from build123d import *

# Parameters (mm, degrees)
BOSS_EXTRUDE1_DEPTH     = 30
BOSS_EXTRUDE2_DEPTH     = 17
SKETCH2_R               = 2
CUT_EXTRUDE7_DEPTH      = 26.5000001
CUT_EXTRUDE2_START      = -17
SKETCH3_R               = 4
CUT_EXTRUDE2_DEPTH      = 9.5000001
CUT_EXTRUDE3_DEPTH      = 31.0000001
CUT_EXTRUDE8_DEPTH      = 6.5
CUT_EXTRUDE8_DEPTH_BACK = 5.6
CHAMFER1_SIZE           = 0.3


with BuildPart() as part:
    # Sketch1 → Boss-Extrude1 (new body)
    with BuildSketch(Plane.XY):
        with BuildLine():
            Line((-9, -10.5), (9, -10.5))
            Line((9, -10.5), (15, -10.5))
            Line((15, -10.5), (15, 0))
            ThreePointArc((15, 0), (0, 15), (-15, 0))
            Line((-15, 0), (-15, -10.5))
            Line((-15, -10.5), (-9, -10.5))
        make_face()
    extrude(amount=BOSS_EXTRUDE1_DEPTH)

    # Sketch4 → Boss-Extrude2 (add)
    with BuildSketch(Plane.XZ.offset(10.5)):
        with BuildLine():
            Line((-12.55, 27.5), (-12.55, 19.5))
            ThreePointArc((-12.55, 19.5), (-16.55, 23.5), (-12.55, 27.5))
        make_face()
        with BuildLine():
            Line((12.55, 2.5), (12.55, 10.5))
            ThreePointArc((12.55, 10.5), (16.55, 6.5), (12.55, 2.5))
        make_face()
    extrude(amount=-BOSS_EXTRUDE2_DEPTH)

    # Sketch2 → Cut-Extrude7 (cut, through all)
    with BuildSketch(Plane.XZ.offset(10.5)):
        with Locations((12.55, 6.5)):
            Circle(SKETCH2_R)
        with Locations((-12.55, 23.5)):
            Circle(SKETCH2_R)
    extrude(amount=-CUT_EXTRUDE7_DEPTH, mode=Mode.SUBTRACT)

    # Sketch3 → Cut-Extrude2 (cut, through all)
    with BuildSketch(Plane.XZ.offset(10.5).offset(CUT_EXTRUDE2_START)):
        with Locations((12.55, 6.5)):
            Circle(SKETCH3_R)
        with Locations((-12.55, 23.5)):
            Circle(SKETCH3_R)
    extrude(amount=-CUT_EXTRUDE2_DEPTH, mode=Mode.SUBTRACT)

    # Sketch5 → Cut-Extrude3 (cut, through all)
    with BuildSketch(Plane.XY.offset(30)):
        with BuildLine():
            Line((-9, -10.5), (9, -10.5))
            Line((9, -10.5), (9, -5.6))
            ThreePointArc((9, -5.6), (0, 10.6), (-9, -5.6))
            Line((-9, -5.6), (-9, -10.5))
        make_face()
    extrude(amount=-CUT_EXTRUDE3_DEPTH, mode=Mode.SUBTRACT)

    # Sketch6 → Cut-Extrude8 (cut, two sides)
    with BuildSketch(Plane(origin=(0, 0, 0), x_dir=(1, 0, 0), z_dir=(0, 1, 0))) as cut_extrude8_sk:
        Polygon((0, -24.914213562), (0, -21.5), (-12.55, -21.5), (-13.964213562, -24.914213562), (-9, -29.878427125), align=None)
        Polygon((0, -7.914213562), (0, -4.5), (12.55, -4.5), (13.964213562, -7.914213562), (9, -12.878427125), align=None)
    extrude(amount=CUT_EXTRUDE8_DEPTH, mode=Mode.SUBTRACT)
    extrude(cut_extrude8_sk.sketch, amount=-CUT_EXTRUDE8_DEPTH_BACK, mode=Mode.SUBTRACT)

    # Chamfer1
    chamfer1_edges = [part.edges().sort_by_distance(p)[0] for p in [
        (0, 15, 0),
        (15, -5.25, 0),
        (-12, -10.5, 0),
        (-15, -5.25, 0),
        (12, -10.5, 0),
        (0, 10.6, 0),
        (9, -8.05, 0),
        (-9, -8.05, 0),
    ]]
    chamfer(chamfer1_edges, length=CHAMFER1_SIZE)


solid = part.part
Verification items for the finished model (mm, model axes). A direction names the side the tool comes from. Round coordinates to 2 decimals unless told otherwise and drop trailing zeros. Loops run counter-clockwise (first coordinate to the right, second up) from the corner with the lowest first, then second, coordinate; pieces in that order, holes last. Notation, with made-up numbers: (84, 59.5) - (109, 59.5) arc R29 cw to (109, 98.5) - close; hole circle Ø2 at (40, 33.25). An arc over 180 degrees is marked (long way). Use one line per item in the form item = value.
1. Scan lines: probe 1 along X at (y, z) = (-8.5, 19); probe 2 along Y at (x, z) = (12, 13); probe 3 along X at (y, z) = (-3, 6.5). Record each from-to range of solid material in increasing order.
A:
probe_1 = -15 to -9, 9 to 15
probe_2 = -10.5 to 9
probe_3 = -15 to -10.17, 14.55 to 16.55
2. Access from +Z, -Z, +X, -X, +Y, -Y to the whole of each face (thin tool, end or side, straight path). Record for faces 4 (the flat face through (-12, -10.5, 15)), 5 (the flat face through (-10, -5.6, 26)), 6 (the flat face through (-15, -5, 10)), 7 (the cylindrical face through (14.397, -4.008, 5.734)), 8 (the flat face through (9, -8, 15)).
A:
face_4 = +Z, -Z, +X, -X, -Y
face_5 = none
face_6 = -Z, -X, +Y, -Y
face_7 = +Y, -Y
face_8 = +Z, -Z, -Y
3. Section check C-C on x = 10. Give the number of separate pieces and of enclosed holes in the cut face, and give its area (3 significant figures).
A:
separate_pieces = 3
enclosed_holes = 0
area = 373 mm²
4. Section check B-B on x = 0. Record the cut outline in (y, z), and give its area (3 significant figures).
A:
outline = (10.6, 0.3) - (10.9, 0) - (14.7, 0) - (15, 0.3) - (15, 30) - (10.6, 30) - close
area = 132 mm²
5. Gauge pin test, flat ends, axial feed: pin 1 Ø1 at (y, z) = (-6, 28) entering from -X; pin 2 Ø3.5 at (y, z) = (-4, 2) entering from +X; pin 3 Ø5.5 at (x, z) = (11.5, 9) entering from +Y. Record the tip position at first contact, or that the pin passes through.
A:
pin_1 = -15
pin_2 = 15.45
pin_3 = 12.18
6. Draft check along Y on faces 1 (the flat face through (15, -5, 20)), 2 (the conical face through (0.326, 14.811, 0.115)), 3 (the cylindrical face through (0.316, 10.595, 15.358)). Enter one of: pulls with the +Y half, pulls with the -Y half, needs draft (parallel to the pull), parting line crosses it, or undercut.
A:
face_1 = needs draft
face_2 = pulls with the +Y half
face_3 = undercut
7. Section check A-A on z = 14. Record the cut outline in (x, y), and give its area (3 significant figures).
A:
outline = (-15, -10.5) - (-9, -10.5) - (-9, -5.6) arc R10.6 cw (long way) to (9, -5.6) - (9, -10.5) - (15, -10.5) - (15, 0) arc R15 ccw to (-15, 0) - close
area = 291 mm²
